Verification items for the finished model (mm, model axes). Coordinates: 2 decimals unless noted, no trailing zeros. Order: outer loops, then holes, each group sorted by start corner. A loop starts at its lowest first (then second) coordinate and runs counter-clockwise, first axis right, second up. Notation, with made-up numbers: (-30, -33) -> (2, -33) arc R30 cw to (2, -7) -> close; hole circle Ø6 at (13.25, 53.25). An arc over 180 degrees is marked (long way). Write item = value, one per line. Start each with the question number.
1. Go/stop test with flat-tipped pins: P1, Ø1.5, axis at y = 29.5, z = 2, coming from the +X side; P2, Ø3, axis at x = 0, y = 44.65, coming from the -Z side; P3, Ø1.5, axis at x = 58.5, z = 2, coming from the -Y side; P4, Ø1.5, axis at y = 31, z = 1, coming from the -X side. Record where each tip stops, or that it passes through.
2. Cross-section at C-C on z = 1.45. Give the number of separate pieces and of enclosed holes in the cut face, plus the area to 3 significant figures.
3. Cross-section at A-A on y = -46. Record the cut outline in (x, z).
4. Thickness scan on line 1 along X through (y, z) = (-8, 1.3); line 2 along Y through (x, z) = (37.5, 1.75); line 3 along Y through (x, z) = (-47.5, 1.05). Record the ranges inside material, lowest first. Write a range as from..to.
5. Cross-section at B-B on x = -47.5. Record the cut outline in (y, z), plus the area to 3 significant figures.
Autodesk Inventor part; units mm, degrees
ref_plane "YZ Plane" through (0, 0, 0) normal (1, 0, 0) x (0, 1, 0)
ref_plane "XZ Plane" through (0, 0, 0) normal (0, 1, 0) x (-1, 0, 0)
ref_plane "XY Plane" through (0, 0, 0) normal (0, 0, 1) x (1, 0, 0)
sketch "Sketch1" plane through (0, 0, 0) normal (0, 0, 1) x (1, 0, 0)
  line L0 (-60, -75) -> (-60, 75)
  line L1 (-60, 75) -> (60, 75)
  line L2 (60, 75) -> (60, -75)
  ellipse E0 centre (0, 72.8464) end of major axis (0, 73.8464) minor radius 1
  line L3 (-6.15, 70.0964) -> (6.15, 70.0964)
  line L4 (6.15, 70.0964) -> (6.15, 47.3964)
  line L5 (6.15, 47.3964) -> (-6.15, 47.3964)
  line L6 (-6.15, 47.3964) -> (-6.15, 70.0964)
  circle A0 centre (0, 44.6464) radius 1
  line L7 (60, 35) -> (57, 35)
  line L8 (57, 35) -> (57, 25)
  line L9 (57, 25) -> (60, 25)
  line L10 (60, 25) -> (60, 35)
  line L11 (37.9, 35) -> (34.9, 35)
  line L12 (34.9, 35) -> (34.9, 25)
  line L13 (34.9, 25) -> (37.9, 25)
  line L14 (37.9, 25) -> (37.9, 35)
  line L15 (-60, 35) -> (-57, 35)
  line L16 (-57, 35) -> (-57, 25)
  line L17 (-57, 25) -> (-60, 25)
  line L18 (-60, 25) -> (-60, 35)
  line L19 (-37.9, 35) -> (-34.9, 35)
  line L20 (-34.9, 35) -> (-34.9, 25)
  line L21 (-34.9, 25) -> (-37.9, 25)
  line L22 (-37.9, 25) -> (-37.9, 35)
  line L23 (-0.5, 73.7124) -> (-0.5, 74.9964)
  line L24 (-0.5, 74.9964) -> (-6.15, 74.9964)
  line L25 (-6.15, 70.0964) -> (-6.15, 74.9964)
  line L26 (6.15, 70.0964) -> (-6.15, 70.0964)
  line L27 (6.15, 70.0964) -> (6.15, 74.9964)
  line L28 (6.15, 74.9964) -> (0.5, 74.9964)
  line L29 (0.5, 74.9964) -> (0.5, 73.7124)
  ellipse E1 centre (0, 72.8464) end of major axis (0, 71.8464) minor radius 1 (-0.5, 73.7124) -> (0.5, 73.7124) ccw
  line L30 (-0.5, 42.4964) -> (-0.5, 43.7803)
  ellipse E2 centre (0, 44.6464) end of major axis (0, 43.6464) minor radius 1 (0.5, 43.7803) -> (-0.5, 43.7803) ccw
  line L31 (0.5, 43.7803) -> (0.5, 42.4964)
  line L32 (6.15, 42.4964) -> (0.5, 42.4964)
  line L33 (6.15, 47.3964) -> (6.15, 42.4964)
  line L34 (-6.15, 47.3964) -> (6.15, 47.3964)
  line L35 (-6.15, 47.3964) -> (-6.15, 42.4964)
  line L36 (-0.5, 42.4964) -> (-6.15, 42.4964)
  line L37 (-6.15, 63.9464) -> (-6.15, 47.3964)
  line L38 (-6.15, 47.3964) -> (6.15, 47.3964)
  line L39 (6.15, 47.3964) -> (6.15, 63.9464)
  line L40 (6.15, 63.9464) -> (6.15, 70.0964)
  line L41 (6.15, 70.0964) -> (0, 70.0964)
  line L42 (0, 70.0964) -> (-6.15, 70.0964)
  line L43 (-6.15, 70.0964) -> (-6.15, 63.9464)
  line L44 (24.5, 3) -> (-24.5, 3)
  line L45 (-24.5, 3) -> (-24.5, 40)
  line L46 (-24.5, 40) -> (24.5, 40)
  line L47 (24.5, 40) -> (24.5, 3)
  circle A1 centre (-18, 21.5) radius 1
  circle A2 centre (18, 21.5) radius 1
  line L48 (19, -46) -> (-19, -46)
  line L49 (-19, -46) -> (-19, -8)
  line L50 (-19, -8) -> (19, -8)
  line L51 (19, -8) -> (19, -46)
  line L52 (19, -46) -> (-19, -8) construction
  line L53 (-19, -46) -> (19, -8) construction
  line L54 (22, -49) -> (-22, -49)
  line L55 (-22, -49) -> (-22, -5)
  line L56 (-22, -5) -> (22, -5)
  line L57 (22, -5) -> (22, -49)
  line L58 (22, -49) -> (-22, -5) construction
  line L59 (-22, -49) -> (22, -5) construction
  line L60 (-22, -5) -> (22, -5)
  line L61 (22, -5) -> (22, -2)
  line L62 (22, -2) -> (-22, -2)
  line L63 (-22, -2) -> (-22, -5)
  circle A3 centre (-19, -8) radius 1.75
  circle A4 centre (19, -8) radius 1.75
  circle A5 centre (-19, -46) radius 1.75
  circle A6 centre (19, -46) radius 1.75
  line L64 (-57, 65) -> (-38, 65)
  line L65 (-38, 65) -> (-38, 0.5)
  line L66 (-38, 0.5) -> (-57, 0.5)
  line L67 (-57, 0.5) -> (-57, 65)
  circle A7 centre (-47.5, -21.7) radius 5
  circle A8 centre (47.5, -21.7) radius 5
  circle A9 centre (0, -57) radius 3
  line L68 (60, -61) -> (60, -80)
  line L69 (60, -80) -> (-60, -80)
  line L70 (-60, -80) -> (-60, -62.9398)
  point P0 (0, 0)
  point P1 (-6.15, 70.0964)
  point P2 (0, -27)
  point P3 (0, -27)
  dimension "d114" = 1
  dimension "d115" = 1
  dimension "d116" = 1
  dimension "d117" = 1
  dimension "d118" = 1
  dimension "d0" = 120
  dimension "d1" = 150
  dimension "d2" = 3
  dimension "d3" = 10
  dimension "d4" = 40
  dimension "d5" = 3
  dimension "d6" = 19.1
  dimension "d7" = 3
  dimension "d8" = 10
  dimension "d9" = 3
  dimension "d10" = 19.1
  dimension "d94" = 49
  dimension "d95" = 37
  dimension "d96" = 32.5036
  dimension "d98" = 35
  dimension "d99" = 2
  dimension "d100" = 2
  dimension "d101" = 36
  dimension "d102" = 6.5
  dimension "d103" = 6.5
  dimension "d104" = 18.5
  dimension "d105" = 18.5
  dimension "d113" = 72
  dimension "d119" = 90
  dimension "d120" = 90
  dimension "d121" = 90
  dimension "d122" = 90
  dimension "d123" = 90
  dimension "d124" = 90
  dimension "d125" = 90
  dimension "d126" = 90
  dimension "d127" = 90
  dimension "d128" = 90
  dimension "d129" = 35.5
  dimension "d130" = 53.85
  dimension "d131" = 53.85
  dimension "d132" = 59.5
  dimension "d133" = 59.5
  dimension "d134" = 60.5
  dimension "d135" = 66.15
  dimension "d136" = 66.15
  dimension "d137" = 94.9
  dimension "d138" = 0
  dimension "d139" = 10
  dimension "d140" = 39.9964
  dimension "d141" = 35.0964
  dimension "d142" = 12.3964
  dimension "d143" = 35.0964
  dimension "d145" = 39.9964
  dimension "d146" = 7.4964
  dimension "d147" = 12.3964
  dimension "d148" = 0
  dimension "d149" = 60
  dimension "d150" = 35
  dimension "d151" = 70.0964
  dimension "d152" = 6.15
  dimension "d153" = 6.15
  dimension "d154" = 6.15
  dimension "d155" = 0.5
  dimension "d156" = 70.0964
  dimension "d157" = 6.15
  dimension "d158" = 47.3964
  dimension "d159" = 6.15
  dimension "d160" = 6.15
extrude "Extrusion1" add sketch "Sketch1" along normal blind 3 contours L0 L17 L67 L66 L65 L64 L15 L1 L2 L7 L8 L9 L68 L69 L70 | L16 L67 L64 L65 L66 | E0 L29 L28 L27 L3 L25 L24 L23 | L5 L33 L32 L31 A0 L30 L36 L35 | L44 L45 L46 L47 | A5 L49 A3 L50 A4 L51 A6 L48 | L54 L55 L56 L57 | L56 L63 L62 L61
fillet "Fillet1" radius 20 4 edges at (-60, 75, 1.5) (60, 75, 1.5) (-60, -80, 1.5) (60, -80, 1.5)
properties part number "Base SD Serayu"
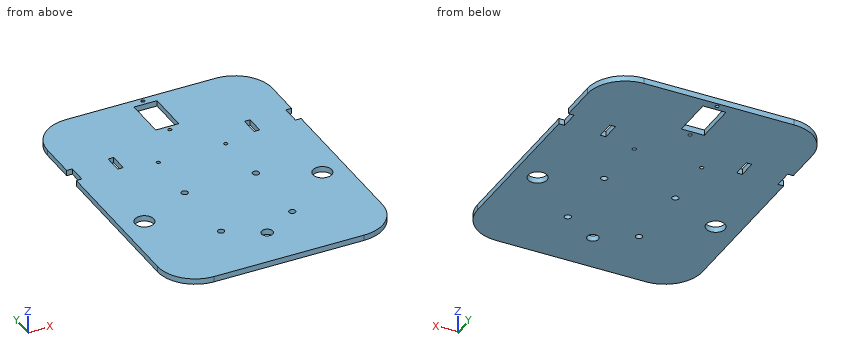
Worked out:
q1.P1 = 57
q1.P2 = 0
q1.P3 = -69.22
q1.P4 = -57
q2.separate_pieces = 1
q2.enclosed_holes = 14
q2.area = 17,600 mm²
q3.outline = (-60, 0) -> (-20.75, 0) -> (-20.75, 3) -> (-60, 3) -> close; (-17.25, 0) -> (17.25, 0) -> (17.25, 3) -> (-17.25, 3) -> close; (20.75, 0) -> (60, 0) -> (60, 3) -> (20.75, 3) -> close
q4.line_1 = -60..-20.75, -17.25..17.25, 20.75..60
q4.line_2 = -80..25, 35..75
q4.line_3 = -78.54..-26.7, -16.7..73.54
q5.outline = (-78.54, 0) -> (-26.7, 0) -> (-26.7, 3) -> (-78.54, 3) -> close; (-16.7, 0) -> (73.54, 0) -> (73.54, 3) -> (-16.7, 3) -> close
q5.area = 426 mm²
